```python
from build123d import *

# Parameters (mm, degrees)
SKETCH1_R           = 11.8618
SKETCH1_R_2         = 0.889
BOSS_EXTRUDE1_DEPTH = 1.778
SKETCH2_R           = 3.4417
SKETCH2_R_2         = 2.19075
BOSS_EXTRUDE2_DEPTH = 3.048
CUT_EXTRUDE1_START  = -1.0922
SKETCH3_R           = 2.159
SKETCH3_R_2         = 0.889
CUT_EXTRUDE1_DEPTH  = 1.0922
SKETCH4_R           = 0.5334
CUT_EXTRUDE2_DEPTH  = 18.455511292


with BuildPart() as part:
    # Sketch1 → Boss-Extrude1 (new body)
    with BuildSketch(Plane(origin=(0, 0, 0), x_dir=(1, 0, 0), z_dir=(0, 1, 0))):
        with Locations(Location((0, 0, 0), (0, 0, 270))):
            Circle(SKETCH1_R)
        with Locations(Location((0, 0, 0), (0, 0, 270))):
            Circle(SKETCH1_R_2, mode=Mode.SUBTRACT)
    extrude(amount=BOSS_EXTRUDE1_DEPTH)

    # Sketch2 → Boss-Extrude2 (add)
    with BuildSketch(Plane.XZ):
        with Locations(Location((0, 0, 0), (0, 0, 90))):
            Circle(SKETCH2_R)
        with Locations(Location((0, 0, 0), (0, 0, 90))):
            Circle(SKETCH2_R_2, mode=Mode.SUBTRACT)
    extrude(amount=BOSS_EXTRUDE2_DEPTH)

    # Sketch3 → Cut-Extrude1 (cut)
    with BuildSketch(Plane(origin=(0, 1.778, 0), x_dir=(1, 0, 0), z_dir=(0, 1, 0)).offset(CUT_EXTRUDE1_START)):
        with Locations(Location((0, 0, 0), (0, 0, 270))):
            Circle(SKETCH3_R)
        with Locations(Location((0, 0, 0), (0, 0, 270))):
            Circle(SKETCH3_R_2, mode=Mode.SUBTRACT)
    extrude(amount=CUT_EXTRUDE1_DEPTH, mode=Mode.SUBTRACT)

    # Sketch4 → Cut-Extrude2 (cut, through all)
    with BuildSketch(Plane(origin=(0, 1.778, 0), x_dir=(1, 0, 0), z_dir=(0, 1, 0))):
        with Locations(Location((0, 9.4742, 0), (0, 0, 270))):
            Circle(SKETCH4_R)
        with Locations(Location((10.414, 0, 0), (0, 0, 270))):
            Circle(SKETCH4_R)
        with Locations(Location((8.3058, 0, 0), (0, 0, 270))):
            Circle(SKETCH4_R)
        with Locations(Location((3.425780113, 8.833147585, 0), (0, 0, 270))):
            Circle(SKETCH4_R)
        with Locations(Location((-3.425780113, 8.833147585, 0), (0, 0, 270))):
            Circle(SKETCH4_R)
        with Locations(Location((7.743695028, 3.003581354, 0), (0, 0, 270))):
            Circle(SKETCH4_R)
        with Locations(Location((9.709220066, 3.765958273, 0), (0, 0, 270))):
            Circle(SKETCH4_R)
        with Locations(Location((7.743695028, -3.003581354, 0), (0, 0, 270))):
            Circle(SKETCH4_R)
        with Locations(Location((9.709220066, -3.765958273, 0), (0, 0, 270))):
            Circle(SKETCH4_R)
        with Locations(Location((3.425780113, -8.833147585, 0), (0, 0, 270))):
            Circle(SKETCH4_R)
        with Locations(Location((0, -9.4742, 0), (0, 0, 270))):
            Circle(SKETCH4_R)
        with Locations(Location((-3.425780113, -8.833147585, 0), (0, 0, 270))):
            Circle(SKETCH4_R)
        with Locations(Location((-9.709220066, -3.765958273, 0), (0, 0, 270))):
            Circle(SKETCH4_R)
        with Locations(Location((-7.743695028, -3.003581354, 0), (0, 0, 270))):
            Circle(SKETCH4_R)
        with Locations(Location((-9.709220066, 3.765958273, 0), (0, 0, 270))):
            Circle(SKETCH4_R)
        with Locations(Location((-7.743695028, 3.003581354, 0), (0, 0, 270))):
            Circle(SKETCH4_R)
        with Locations(Location((-8.3058, 0, 0), (0, 0, 270))):
            Circle(SKETCH4_R)
        with Locations(Location((-10.414, 0, 0), (0, 0, 270))):
            Circle(SKETCH4_R)
    extrude(amount=-CUT_EXTRUDE2_DEPTH, mode=Mode.SUBTRACT)


solid = part.part
```
The listing builds one solid part. Answer for the finished solid, in the listing's coordinates (mm). A direction names the side the tool comes from. Round coordinates to 2 decimals unless told otherwise and drop trailing zeros. Order: outer loops, then holes, each group sorted by start corner. A loop starts at its lowest first (then second) coordinate and runs counter-clockwise, first axis right, second up. Notation, with made-up numbers: (-19.5, 17) -> (-11.5, 17) arc R16 ccw to (-11.5, 29) -> close; hole circle Ø10 at (70.5, 8). An arc over 180 degrees is marked (long way). Answer as CSV lines item,"result". Start each with the question number.
(1) For a pull along X with two mould halves and no side action, classify faces 1 (the face through (2.094, -1.503, -2.731)), 2 (the face through (-3.402, 0.901, -9.366)), 3 (the face through (-2.5, 1.778, -0.2)) as +X half, -X half, draft (parallel to the pull), parting line (faces both ways), or undercut.
(2) The part is cut by section D-D (x = 5.5). Determine the outline of the cut face in (y, z), then the cut area to 3 significant figures.
(3) Find the intervals of material crossed by probe 1 along X at (y, z) = (0.95, 9.25); probe 2 along Y at (x, z) = (0.75, 8.25); probe 3 along Z at (x, y) = (7.5, 1.5), in increasing order. Write a range as from..to.
(4) Flat-ended cylindrical pins translate along their axes: pin 1 Ø1.4 at (x, z) = (0, 9.47) entering from -Y; pin 2 Ø2.5 at (x, z) = (0, 0) entering from +Y; pin 3 Ø12 at (x, z) = (-0.5, -0.5) entering from -Y; pin 4 Ø2 at (x, y) = (-3.5, -2) entering from -Z. Find the tip coordinate at first contact, or state that the pin passes through.
(5) The part is cut by section C-C (z = 0). Count the separate pieces of the cut face and the enclosed holes in it, then the cut area to 3 significant figures.
(6) The part is cut by section A-A (x = 0). Determine the outline of the cut face in (y, z).
(7) The part is cut by section B-B (y = -1.65). Determine the outline of the cut face in (x, z).
(8) A tool of negligible diameter and unlimited length cuts with its end or side. For faces 4 (the face through (-0.46, 0, 0.94)), 5 (the face through (-10.23, 0.9, -3.88)), from which of +Z, -Z, +X, -X, +Y, -Y can it reach the whole face along a straight path? Write none if from no direction.
Evaluation:
1,face 1,"parting line"
1,face 2,"undercut"
1,face 3,"draft"
2,outline,"(0, -10.51) -> (1.78, -10.51) -> (1.78, 10.51) -> (0, 10.51) -> close"
2,area,"37.4 mm²"
3,probe 1,"-7.43..-3.76, -3.09..-0.48, 0.48..3.09, 3.76..7.43"
3,probe 2,"0..1.78"
3,probe 3,"-9.19..-3.48, -2.53..2.53, 3.48..9.19"
4,pin 1,"y = 0"
4,pin 2,"y = 0.69"
4,pin 3,"y = -3.05"
4,pin 4,"z = -2.37"
5,separate pieces,"6"
5,enclosed holes,"0"
5,area,"36.3 mm²"
6,outline,"(-3.05, -3.44) -> (0, -3.44) -> (0, -8.94) -> (1.78, -8.94) -> (1.78, -2.16) -> (0.69, -2.16) -> (0.69, -0.89) -> (0, -0.89) -> (0, -2.19) -> (-3.05, -2.19) -> close; (-3.05, 2.19) -> (0, 2.19) -> (0, 0.89) -> (0.69, 0.89) -> (0.69, 2.16) -> (1.78, 2.16) -> (1.78, 8.94) -> (0, 8.94) -> (0, 3.44) -> (-3.05, 3.44) -> close; (0, -11.86) -> (1.78, -11.86) -> (1.78, -10.01) -> (0, -10.01) -> close; (0, 10.01) -> (1.78, 10.01) -> (1.78, 11.86) -> (0, 11.86) -> close"
7,outline,"circle Ø6.88 at (0, 0); hole circle Ø4.38 at (0, 0)"
8,face 4,"-Y"
8,face 5,"+Y, -Y"
